Source: CAD feature listing. Evaluate the final solid. Frame: model axes, mm. Face numbers are marked on the shaded views. A direction names the side the tool comes from. Give positions to 0.01 mm unless a question says otherwise; leave off trailing zeros. Write each loop counter-clockwise with the first axis right and the second up, starting at its lowest first coordinate (ties: lowest second). Pieces come first, ordered by that corner, then holes. Notation, with made-up numbers: (83, 84) - (114, 84) arc R10 ccw to (114, 100) - close; hole circle Ø8 at (86.5, 74.25). An arc over 180 degrees is marked (long way). One line per question, with ' | ' between items. Start each with the question number.
(1) Draft query along Z for the marked faces 1, 2 and 3. Return one class per face: +Z half, -Z half, draft (parallel to the pull), parting line (faces both ways), or undercut.
(2) Ray query, line 1 (X direction, y = 5.25, z = 59.5); line 2 (Z direction, x = 2.95, y = 0); line 3 (Y direction, x = 0.5, z = 65). Return the intervals inside material, ascending. Write a range as [from, to].
(3) Section B-B, the plane x = 0. Return loops of the section in (y, z), plus the area to 3 significant figures.
(4) Pin query (flat end, axial travel): pin 1 (6 mm diameter, centred on y = -2, z = 61, fed in from +X); pin 2 (10 mm diameter, centred on x = -7, y = 4.5, fed in from +Z); pin 3 (6 mm diameter, centred on y = 7.5, z = 22, fed in from -X); pin 4 (12 mm diameter, centred on y = -7, z = 66, fed in from -X). Return the tip coordinate at first contact, or that it passes through.
(5) Section D-D, the plane y = 7.5. Return loops of the section in (x, z), plus the area to 3 significant figures.
(6) Section A-A, the plane y = 0. Return loops of the section in (x, z), plus the area to 3 significant figures.
(7) Section C-C, the plane z = 57. Return loops of the section in (x, y).
(8) Access query for the marked faces 4, 5, 6, 7 and 8. Directions: +Z, -Z, +X, -X, +Y, -Y. A direction counts if a zero-diameter tool reaches every point of the face in a straight line with its end or side. Return the directions, or none.
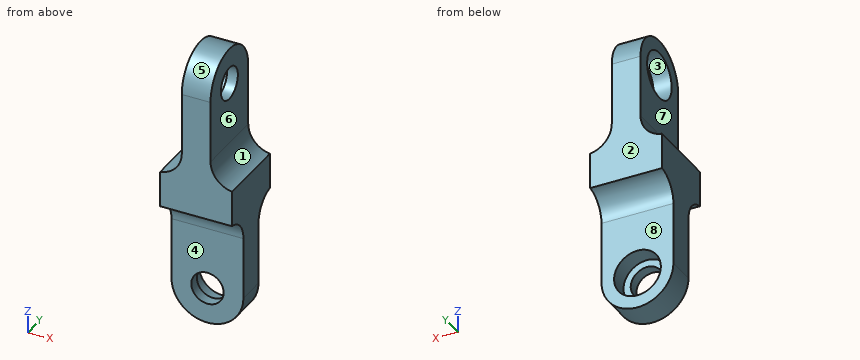
```python
from build123d import *

# Parameters (mm, degrees)
SKETCH_1_W          = 20
SKETCH_1_H          = 20
EXTRUDE_1_DEPTH     = 80.297387422
SKETCH_7_W          = 35.148693711
SKETCH_7_H          = 6
CUT_EXTRUDE_6_DEPTH = 34
SKETCH_2_R          = 6.5
CUT_EXTRUDE_9_DEPTH = 5
SKETCH_3_R          = 4.5
CUT_EXTRUDE_2_DEPTH = 29
MOVE_BODY_1_ANGLE   = 90
SKETCH_8_W          = 20
SKETCH_8_H          = 20
EXTRUDE_2_DEPTH     = 8
FILLET_2_R          = 7


# Read off the part's stored shape, not the designer's step: the other step
with BuildPart() as part:
    # Sketch 1 → Extrude 1 (new body)
    with BuildSketch(Plane.XY):
        Rectangle(SKETCH_1_W, SKETCH_1_H)
    extrude(amount=EXTRUDE_1_DEPTH)

    # Sketch 7 → Cut-Extrude 6 (cut)
    with BuildSketch(Plane(origin=(10, 0, 0), x_dir=(0, 0, -1), z_dir=(1, 0, 0))):
        with Locations((-17.574346855, 7)):
            Rectangle(SKETCH_7_W, SKETCH_7_H)
        with Locations((-17.574346855, -7)):
            Rectangle(SKETCH_7_W, SKETCH_7_H)
    cut_extrude_6 = extrude(amount=-CUT_EXTRUDE_6_DEPTH, mode=Mode.SUBTRACT)

    # Sketch 2 → Cut-Extrude 9 (cut)
    with BuildSketch(Plane(origin=(0, 4, 0), x_dir=(-1, 0, 0), z_dir=(0, -1, 0))):
        with Locations(Location((0, -10.902706153, 0), (0, 0, 90))):
            Circle(SKETCH_2_R)
    cut_extrude_9 = extrude(amount=CUT_EXTRUDE_9_DEPTH, mode=Mode.SUBTRACT)

    # Sketch 3 → Cut-Extrude 2 (cut)
    with BuildSketch(Plane(origin=(0, -4, 0), x_dir=(-1, 0, 0), z_dir=(0, -1, 0))):
        with Locations(Location((0, -10.902706153, 0), (0, 0, 90))):
            Circle(SKETCH_3_R)
        with BuildLine():
            Line((-21.262122506, -10.902706153), (-10, -10.902706153))
            ThreePointArc((-10, -10.902706153), (0, -0.902706153), (10, -10.902706153))
            Line((10, -10.902706153), (21.262122506, -10.902706153))
            ThreePointArc((21.262122506, -10.902706153), (0, 10.359416353), (-21.262122506, -10.902706153))
        make_face()
    cut_extrude_2 = extrude(amount=-CUT_EXTRUDE_2_DEPTH, mode=Mode.SUBTRACT)

    # Mirror 6: Cut-Extrude 6, Cut-Extrude 9, Cut-Extrude 2 across plane
    add(cut_extrude_6.mirror(Plane.XY.offset(40.148693711)), mode=Mode.SUBTRACT)
    add(cut_extrude_9.mirror(Plane.XY.offset(40.148693711)), mode=Mode.SUBTRACT)
    add(cut_extrude_2.mirror(Plane.XY.offset(40.148693711)), mode=Mode.SUBTRACT)


with BuildPart() as body_2:
    # Other 3: the piece on the far side of the plane
    add(part.part)
    split(bisect_by=Plane.XY.offset(40.148693711), keep=Keep.BOTTOM)


with BuildPart() as part_1:
    add(part.part)

    # Other 3
    split(bisect_by=Plane.XY.offset(40.148693711), keep=Keep.TOP)


with BuildPart() as part_2:
    # Move Body 1: moved
    add(part_1.part.rotate(Axis((0, 0, 0), (0, 0, 1)), MOVE_BODY_1_ANGLE))


    add(body_2.part)  # Extrude 2 merges body 2
    # Sketch 8 → Extrude 2 (add)
    with BuildSketch(Plane.XY.offset(45.148693711)):
        Rectangle(SKETCH_8_W, SKETCH_8_H)
    extrude(amount=-EXTRUDE_2_DEPTH)

    # Fillet 2
    # the kernel refuses this fillet: 7 mm, written as the material it adds along each edge
    with BuildSketch(Plane(origin=(-4, 10, 45.148693711), x_dir=(0, 0, 1), z_dir=(0, -1, 0)), Plane(origin=(10, -4, 35.148693711), x_dir=(0, 0, -1), z_dir=(-1, 0, 0))) as fillet_2_piece_1:
        with BuildLine():
            CenterArc((6.92820323, 7), FILLET_2_R, 188.213210702, 81.786789298)
            Line((0, 6), (-0.138564065, 5.98))
            ThreePointArc((-0.138564065, 5.98), (-0.14, 3), (-0.14, 0))
            Line((-0.14, 0), (0, -0.14))
            Line((0, -0.14), (6.92820323, -0.14))
            Line((6.92820323, -0.14), (6.92820323, 0))
        make_face()
    extrude(amount=20)
    with BuildSketch(Plane(origin=(4, 10, 45.148693711), x_dir=(1, 0, 0), z_dir=(0, -1, 0))) as fillet_2_piece_2:
        with BuildLine():
            CenterArc((7, 6.92820323), FILLET_2_R, 180, 81.786789298)
            Line((0, 6.92820323), (-0.14, 6.92820323))
            Line((-0.14, 6.92820323), (-0.14, 0))
            Line((-0.14, 0), (0, -0.14))
            ThreePointArc((0, -0.14), (3, -0.14), (5.98, -0.138564065))
            Line((5.98, -0.138564065), (6, 0))
        make_face()
    extrude(amount=20)
    with BuildSketch(Plane(origin=(10, 4, 35.148693711), x_dir=(0, 0, -1), z_dir=(-1, 0, 0))) as fillet_2_piece_3:
        with BuildLine():
            CenterArc((6.92820323, -7), FILLET_2_R, 90, 81.786789298)
            Line((0, -6), (-0.138564065, -5.98))
            ThreePointArc((-0.138564065, -5.98), (-0.14, -3), (-0.14, 0))
            Line((-0.14, 0), (0, 0.14))
            Line((0, 0.14), (6.92820323, 0.14))
            Line((6.92820323, 0.14), (6.92820323, 0))
        make_face()
    extrude(amount=20)


solid = part_2.part
```
Check sheet entries:
1) face 1: +Z half | face 2: draft | face 3: undercut
2) line 1: [-4, 4] | line 2: [1.35, 5.11], [16.69, 64.89], [73.89, 79.39] | line 3: [-10, -4.79], [4.79, 10]
3) outline: (-10, 35.15) arc R7 cw to (-4, 28.22) - (-4, 15.4) - (-1, 15.4) - (-1, 17.4) - (4, 17.4) - (4, 28.22) arc R7 cw to (10, 35.15) - (10, 69.39) arc R10 ccw to (-10, 69.39) - close; (-4, 0.9) - (4, 0.9) - (4, 4.4) - (-1, 4.4) - (-1, 6.4) - (-4, 6.4) - close; hole circle Ø13 at (0, 69.39) | area: 911 mm²
4) pin 1: x = 4 | pin 2: z = 79.38 | pin 3: through | pin 4: x = -4
5) outline: (-10, 34.28) - (10, 34.28) - (10, 45.15) arc R7 cw to (4, 52.08) - (4, 76.01) - (-4, 76.01) - (-4, 52.08) arc R7 cw to (-10, 45.15) - close | area: 484 mm²
6) outline: (-10, 10.9) arc R10 ccw to (10, 10.9) - (10, 45.15) arc R7 cw to (4, 52.08) - (4, 64.89) - (1, 64.89) - (1, 62.89) - (-4, 62.89) - (-4, 52.08) arc R7 cw to (-10, 45.15) - close; (-4, 75.89) - (1, 75.89) - (1, 73.89) - (4, 73.89) - (4, 79.39) - (-4, 79.39) - close; hole circle Ø13 at (0, 10.9) | area: 911 mm²
7) outline: (-4, -10) - (4, -10) - (4, 10) - (-4, 10) - close
8) face 4: -Z, +X, -X, -Y | face 5: +Z, +X, -X | face 6: +Z, +X, +Y, -Y | face 7: +Z, -X, +Y, -Y | face 8: -Z, +X, -X, +Y
